```python
from build123d import *

# Parameters (mm, degrees)
SKETCH1_R          = 6.35
EXTRUDE1_DEPTH     = 25.4
CUT_EXTRUDE1_DEPTH = 6.35
FILLET1_R          = 3.175


with BuildPart() as part:
    # Sketch1 → Extrude1 (new body)
    with BuildSketch(Plane.XY):
        with Locations((-109.908874461, 962.175)):
            Circle(SKETCH1_R)
    extrude(amount=-EXTRUDE1_DEPTH)

    # Sketch2 → Cut-Extrude1 (cut)
    with BuildSketch(Plane(origin=(0, 0, -6.35), x_dir=(-1, 0, 0), z_dir=(0, 0, -1))):
        with BuildLine():
            ThreePointArc((111.178874461, 968.396703947), (106.098874461, 962.175), (111.178874461, 955.953296053))
            ThreePointArc((111.178874461, 955.953296053), (103.558874461, 962.175), (111.178874461, 968.396703947))
        make_face()
    extrude(amount=CUT_EXTRUDE1_DEPTH, mode=Mode.SUBTRACT)

    # Fillet1
    fillet1_edges = [part.edges().sort_by_distance(p)[0] for p in [
        (-116.258874461, 962.175, -25.4),
    ]]
    fillet(fillet1_edges, radius=FILLET1_R)


solid = part.part
```
For this review, take the finished solid that the model builds, in its own axes (mm). A direction names the side the tool comes from. Coordinates: 2 decimals unless noted, no trailing zeros. Order: outer loops, then holes, each group sorted by start corner. A loop starts at its lowest first (then second) coordinate and runs counter-clockwise, first axis right, second up. Notation, with made-up numbers: (36.5, 51.25) -> (83.5, 51.25) arc R18 cw to (83.5, 67.25) -> close; hole circle Ø8 at (21, -35.75). An arc over 180 degrees is marked (long way). Use CSV: the item, a comma, the result in double quotes. Start each with the question number.
Item 1: We need section A-A, the plane z = -6.75. Give the boundary of the cut face in (x, y) (3 decimals), then the cut area to 3 significant figures.
Item 2: We need section B-B, the plane z = -20. Give the boundary of the cut face in (x, y) (3 decimals).
Item 3: Wall thickness on probe 1 along Z at (x, y) = (-108.25, 957.25); probe 2 along X at (y, z) = (959.5, -15); probe 3 along X at (y, z) = (956.5, -16.5): over which ranges is each line inside the solid? List them lowest first.
Item 4: For faces 1 (the face through (-116.253, 962.454, -10.957)), 2 (the face through (-106.1, 962.3, -9.5)), list the 3-axis set-ups (+Z, -Z, +X, -X, +Y, -Y) from which the entire face can be reached by the end or side of a thin tool; tool diameter is ignored.
Item 5: Draft analysis for pull direction Z (two halves, no side actions). For faces 3 (the face through (-110, 962, -25.4)), 4 (the face through (-105.7, 962.2, -12.7)), 5 (the face through (-105.7, 962.2, -6.35)), 6 (the face through (-110, 962, 0)), state which applies: pulls with the +Z half, pulls with the -Z half, needs draft (parallel to the pull), parting line crosses it, or undercut.
Item 6: Insertion check: pin 1 (1 mm diameter, centred on x = -106.5, z = -22.5, fed in from -Y); pin 2 (3 mm diameter, centred on x = -107, z = -21, fed in from +Y); pin 3 (1.5 mm diameter, centred on x = -114.5, z = -11.5, fed in from -Y). Each pin has a flat end and moves straight along its axis. Give the tip position at first contact, or say it passes through.
Derived:
1,outline,"(-111.179, 955.953) arc R6.35 ccw to (-111.179, 968.397) arc R6.35 ccw to start"
1,area,"94.6 mm^2"
2,outline,"circle Ø12.7 at (-109.909, 962.175)"
3,probe 1,"z = -24.67 to -12.7, -6.35 to 0"
3,probe 2,"x = -115.67 to -104.15"
3,probe 3,"x = -112.76 to -107.06"
4,face 1,"+Z, -Z"
4,face 2,"+X"
5,face 3,"pulls with the -Z half"
5,face 4,"undercut"
5,face 5,"undercut"
5,face 6,"pulls with the +Z half"
6,pin 1,"stops at y = 956.54"
6,pin 2,"stops at y = 968.37"
6,pin 3,"stops at y = 957.12"
